from build123d import *

# Parameters (mm, degrees)
SKETCH1_R           = 3
BOSS_EXTRUDE1_DEPTH = 30
CUT_EXTRUDE1_DEPTH  = 2
CHAMFER1_SIZE       = 0.5


with BuildPart() as part:
    # Sketch1 → Boss-Extrude1 (new body)
    with BuildSketch(Plane(origin=(0, 0, 0), x_dir=(1, 0, 0), z_dir=(0, 1, 0))):
        with Locations(Location((0, 0, 0), (0, 0, 270))):
            Circle(SKETCH1_R)
    extrude(amount=-BOSS_EXTRUDE1_DEPTH)

    # Sketch2 → Cut-Extrude1 (cut)
    with BuildSketch(Plane(origin=(0, 0, 0), x_dir=(1, 0, 0), z_dir=(0, 1, 0))):
        Polygon((0, 1.732050808), (-1.5, 0.866025404), (-1.5, -0.866025404), (0, -1.732050808), (1.5, -0.866025404), (1.5, 0.866025404), align=None)
    extrude(amount=-CUT_EXTRUDE1_DEPTH, mode=Mode.SUBTRACT)

    # Chamfer1
    chamfer1_edges = [part.edges().sort_by_distance(p)[0] for p in [
        (0, 0, -3),
        (0, -30, -3),
    ]]
    chamfer(chamfer1_edges, length=CHAMFER1_SIZE)


solid = part.part
Verification items for the finished model (mm, model axes). A direction names the side the tool comes from. Coordinates: 2 decimals unless noted, no trailing zeros. Order: outer loops, then holes, each group sorted by start corner. A loop starts at its lowest first (then second) coordinate and runs counter-clockwise, first axis right, second up.
1. Sectioned sample at B-B, the plane y = -12.25. Record the cut outline in (x, z), and give its area (3 significant figures).
Results found:
outline: circle Ø6 at (0, 0)
area: 28.3 mm2
2. Go/stop test with a flat-tipped pin: pin 1 Ø0.9 at (x, z) = (0, 0.5) entering from +Y. Record where the tip stops, or that it passes through.
Results found:
pin 1: stops at y = -2
3. Scan lines: line 1 (X direction, y = -5.25, z = -2.45); line 2 (X direction, y = -5.5, z = 2.6); line 3 (Y direction, x = -0.1, z = -0.6). Record each from-to range of solid material in increasing order.
Results found:
line 1: x = -1.73 to 1.73
line 2: x = -1.5 to 1.5
line 3: y = -30 to -2
4. Sectioned sample at A-A, the plane z = 0. Record the cut outline in (x, y), and give its area (4 significant figures).
Results found:
outline: (-3, -29.5) - (-2.5, -30) - (2.5, -30) - (3, -29.5) - (3, -0.5) - (2.5, 0) - (1.5, 0) - (1.5, -2) - (-1.5, -2) - (-1.5, 0) - (-2.5, 0) - (-3, -0.5) - close
area: 173.5 mm2
5. Set-up check for faces 4 (the face through (-2, 0, 0)), 5 (the face through (-1.5, -1, 0)): record each of +Z, -Z, +X, -X, +Y, -Y from which the full face is reachable in a straight line by a thin tool's end or side.
Results found:
face 4: +Z, -Z, +X, -X, +Y
face 5: +Y
6. Release check for a two-part mould opening along X. For faces 1 (the face through (0.9, -14.8, 2.86)), 2 (the face through (0.74, -0.986, 1.305)), 3 (the face through (0, -30, 0)) record: +X half, -X half, draft (parallel to the pull), parting line (faces both ways), or undercut.
Results found:
face 1: parting line
face 2: undercut
face 3: draft
